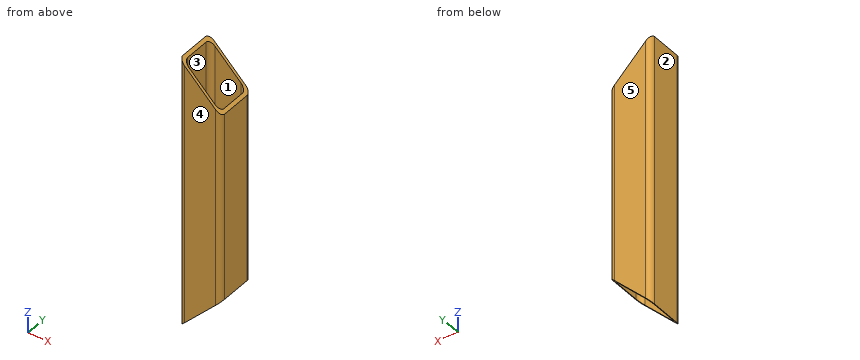
```python
from build123d import *

# Parameters (mm, degrees)
F1_W     = 25.4
F1_H     = 25.4
F2_DEPTH = 165.1
F4_DEPTH = 25.4
F5_R     = 3.175


# Not quite as in the source:
# - a variable given as a bare number and used for a length is read in inches; the dataset says mm whatever the document's units were


with BuildPart() as f2:
    # F1 (on Top) → F2 (new body)
    with BuildSketch(Plane.XY):
        Rectangle(F1_W, F1_H)
        with BuildLine():
            ThreePointArc((-11.049, 7.874), (-10.1190640303, 10.1190640303), (-7.874, 11.049))
            Line((-7.874, 11.049), (7.874, 11.049))
            ThreePointArc((7.874, 11.049), (10.1190640303, 10.1190640303), (11.049, 7.874))
            Line((11.049, 7.874), (11.049, -7.874))
            ThreePointArc((11.049, -7.874), (10.1190640303, -10.1190640303), (7.874, -11.049))
            Line((7.874, -11.049), (-7.874, -11.049))
            ThreePointArc((-7.874, -11.049), (-10.1190640303, -10.1190640303), (-11.049, -7.874))
            Line((-11.049, -7.874), (-11.049, 7.874))
        make_face(mode=Mode.SUBTRACT)
    extrude(amount=F2_DEPTH)

    # F3 (on face) → F4 (cut)
    with BuildSketch(Plane.XZ.offset(12.7)):
        Polygon((12.7, 25.4), (-12.7, 0), (12.7, 0), align=None)
        Polygon((12.7, 165.1), (-12.7, 165.1), (12.7, 139.7), align=None)
    extrude(amount=-F4_DEPTH, mode=Mode.SUBTRACT)

    # F5
    f5_edges = [f2.edges().sort_by_distance(p)[0] for p in [
        (-12.7, 12.7, 82.55),
        (12.7, 12.7, 82.55),
        (-12.7, -12.7, 82.55),
        (12.7, -12.7, 82.55),
    ]]
    fillet(f5_edges, radius=F5_R)


solid = f2.part
```
Can you work these out from the model? Positions are in its coordinate system, mm. Face numbers are marked on the shaded views. A direction names the side the tool comes from. Round coordinates to 2 decimals unless told otherwise and drop trailing zeros. Order: outer loops, then holes, each group sorted by start corner. A loop starts at its lowest first (then second) coordinate and runs counter-clockwise, first axis right, second up.
(1) If we section it at A-A (x = 3): Please give me the cut outline in (y, z), plus the area to 3 significant figures.
Results are:
outline: (-12.7, 15.7) - (-11.05, 15.7) - (-11.05, 149.4) - (-12.7, 149.4) - close; (11.05, 15.7) - (12.7, 15.7) - (12.7, 149.4) - (11.05, 149.4) - close
area: 441 mm2
(2) If we section it at D-D (z = 13.5): Please give me the cut outline in (x, y) (3 decimals), plus the area to 3 significant figures.
Results are:
outline: (-12.7, -9.525) arc R3.175 ccw to (-9.525, -12.7) - (0.8, -12.7) - (0.8, -11.049) - (-7.874, -11.049) arc R3.175 cw to (-11.049, -7.874) - (-11.049, 7.874) arc R3.175 cw to (-7.874, 11.049) - (0.8, 11.049) - (0.8, 12.7) - (-9.525, 12.7) arc R3.175 ccw to (-12.7, 9.525) - close
area: 81.1 mm2
(3) We'd pull the mould along Y, two halves only. Please class the marked faces 3, 4 and 5: +Y half, -Y half, draft (parallel to the pull), parting line (faces both ways), or undercut.
Results are:
face 3: undercut
face 4: -Y half
face 5: +Y half
(4) If we section it at B-B (z = 56): Please give me the cut outline in (x, y) (3 decimals), plus the area to 3 significant figures.
Results are:
outline: (-12.7, -9.525) arc R3.175 ccw to (-9.525, -12.7) - (9.525, -12.7) arc R3.175 ccw to (12.7, -9.525) - (12.7, 9.525) arc R3.175 ccw to (9.525, 12.7) - (-9.525, 12.7) arc R3.175 ccw to (-12.7, 9.525) - close; hole (-11.049, -7.874) arc R3.175 ccw to (-7.874, -11.049) - (7.874, -11.049) arc R3.175 ccw to (11.049, -7.874) - (11.049, 7.874) arc R3.175 ccw to (7.874, 11.049) - (-7.874, 11.049) arc R3.175 ccw to (-11.049, 7.874) - close
area: 157 mm2
(5) If I drill on L1, parallel to X at y = 7.5, z = 127.5; L2, parallel to X at y = -9.75, z = 46.5, over which ranges is the centre line in solid material (lowest first)?
Results are:
L1: x = -12.7 to -11.05, 11.05 to 12.7
L2: x = -12.69 to -10.44, 10.44 to 12.69
(6) If we section it at C-C (y = -3.5): Please give me the cut outline in (x, z).
Results are:
outline: (-12.7, 0) - (-11.05, 1.65) - (-11.05, 163.45) - (-12.7, 165.1) - close; (11.05, 23.75) - (12.7, 25.4) - (12.7, 139.7) - (11.05, 141.35) - close
(7) I'm going to push flat-ended pins straight in: pin 1 (5 mm diameter, centred on x = 10, y = -7.5, fed in from -Z); pin 2 (12 mm diameter, centred on x = 4, y = -9, fed in from +Z). Where does each tip first touch, or does it pass through?
Results are:
pin 1: stops at z = 22.94
pin 2: stops at z = 154.04
(8) On a 3-axis mill with a long thin cutter (end or side, diameter ignored), from which of +Z, -Z, +X, -X, +Y, -Y can I reach the whole of each face in a straight line? I mean the marked faces 1 and 2. Say none if no direction works.
Results are:
face 1: +Z, -Z
face 2: +Z, -Z, -X, +Y, -Y
